Check sheet for the modelled part. Datum: model origin and axes. Units: mm. A direction names the side the tool comes from. Give positions to 0.01 mm unless a question says otherwise; leave off trailing zeros. Write each loop counter-clockwise with the first axis right and the second up, starting at its lowest first coordinate (ties: lowest second). Pieces come first, ordered by that corner, then holes. Notation, with made-up numbers: M 20,61.5 L 51,61.5 A21 cw 51,81.5 Z; hole C 61,43 d3. An arc over 180 degrees is marked long. Write item = value, one per line. Start each with the question number.
1) Draft check along X on faces 3 (the face through (132.08, -2, 0)), 4 (the face through (-47.568, -5, 0)), 5 (the face through (-132.08, -2, 0)), 6 (the face through (-2, 2, -5.08)). Enter one of: pulls with the +X half, pulls with the -X half, needs draft (parallel to the pull), parting line crosses it, or undercut.
2) Sectioned sample at C-C, the plane x = 66.04. Record the cut outline in (y, z) (3 decimals), then the cut area to 3 significant figures.
3) Sectioned sample at A-A, the plane x = -56.5. Record the cut outline in (y, z), then the cut area to 3 significant figures.
4) Scan lines: L1, parallel to Y at x = -46, z = -2.25; L2, parallel to Y at x = -59, z = 3.5; L3, parallel to X at y = 45.5, z = 1. Record each from-to range of solid material in increasing order.
5) Sectioned sample at B-B, the plane z = 0.5. Record the cut outline in (x, y) (3 decimals), then the cut area to 3 significant figures.
6) Set-up check for faces 1 (the face through (-2.54, 56, 0)), 2 (the face through (-2, -132.08, 0)): record each of +Z, -Z, +X, -X, +Y, -Y from which the full face is reachable in a straight line by a thin tool's end or side.
from build123d import *

# Parameters (mm, degrees)
SKETCH1_W           = 264.16
SKETCH1_H           = 264.16
BOSS_EXTRUDE1_DEPTH = 5.08
SKETCH2_R           = 10.16
SKETCH2_W           = 73.66
SKETCH2_H           = 24.13
SKETCH2_W_2         = 19.812
SKETCH2_H_2         = 23.368
CUT_EXTRUDE1_DEPTH  = 11.16


with BuildPart() as part:
    # Sketch1 → Boss-Extrude1 (new body, symmetric)
    with BuildSketch(Plane.XY):
        Rectangle(SKETCH1_W, SKETCH1_H)
    extrude(amount=BOSS_EXTRUDE1_DEPTH, both=True)

    # Sketch2 → Cut-Extrude1 (cut, through all)
    with BuildSketch(Plane.XY.offset(5.08)):
        with Locations((26.67, 56.515)):
            Circle(SKETCH2_R)
        with Locations((66.04, 56.515)):
            Circle(SKETCH2_R)
        with Locations((-39.37, 56.515)):
            Rectangle(SKETCH2_W, SKETCH2_H)
        with Locations((-37.662476274, -5.334)):
            Rectangle(SKETCH2_W_2, SKETCH2_H_2)
    extrude(amount=-CUT_EXTRUDE1_DEPTH, mode=Mode.SUBTRACT)


solid = part.part
Data:
q1.face_3 = pulls with the +X half
q1.face_4 = undercut
q1.face_5 = pulls with the -X half
q1.face_6 = needs draft
q2.outline = M -132.08,-5.08 L 46.355,-5.08 L 46.355,5.08 L -132.08,5.08 Z; M 66.675,-5.08 L 132.08,-5.08 L 132.08,5.08 L 66.675,5.08 Z
q2.area = 2,480 mm2
q3.outline = M -132.08,-5.08 L 44.45,-5.08 L 44.45,5.08 L -132.08,5.08 Z; M 68.58,-5.08 L 132.08,-5.08 L 132.08,5.08 L 68.58,5.08 Z
q3.area = 2,440 mm2
q4.L1 = -132.08 to -17.02, 6.35 to 44.45, 68.58 to 132.08
q4.L2 = -132.08 to 44.45, 68.58 to 132.08
q4.L3 = -132.08 to -76.2, -2.54 to 132.08
q5.outline = M -132.08,-132.08 L 132.08,-132.08 L 132.08,132.08 L -132.08,132.08 Z; hole M -76.2,44.45 L -2.54,44.45 L -2.54,68.58 L -76.2,68.58 Z; hole M -47.568,-17.018 L -27.756,-17.018 L -27.756,6.35 L -47.568,6.35 Z; hole C 26.67,56.515 d20.32; hole C 66.04,56.515 d20.32
q5.area = 66,900 mm2
q6.face_1 = +Z, -Z
q6.face_2 = +Z, -Z, +X, -X, -Y
